Input: part model. Units: mm. Frame: model coordinates. A direction names the side the tool comes from. Give positions to 0.01 mm unless a question says otherwise; leave off trailing zeros. Loops run counter-clockwise (first coordinate to the right, second up) from the corner with the lowest first, then second, coordinate; pieces in that order, holes last.
Autodesk Fusion 360 part; units mm, degrees
sketch "Sketch1" plane through (0, 0, 0) normal (0, 0, 1) x (1, 0, 0)
  circle A0 centre (0, 0) radius 5.25
  circle A1 centre (0, 0) radius 3.1
  circle A2 centre (0, 0) radius 1.85
  circle A3 centre (0, 0) radius 3.4
  circle A4 centre (0, 0) radius 1.55
  dimension "d1" = 10.5
  dimension "d2" = 6.2
  dimension "d3" = 3.7
  dimension "d21" = 0.3
  dimension "d22" = 0.3
extrude "Extrude1" add sketch "Sketch1" along normal blind 9.5 contours A1
extrude "Extrude2" add sketch "Sketch1" along normal blind 2 contours A0 | A3
extrude "Extrude3" add sketch "Sketch1" along normal blind 4 and the other way blind -5 contours A3
chamfer "Chamfer1" distance 0.2 angle 45 2 edges at (-3.1699, -1.2295, 4) (-3.1699, -1.2295, 5)
chamfer "Chamfer2" distance 0.5 angle 45 1 edges at (-1.7248, 0.669, 0)
extrude "Extrude4" add sketch "Sketch1" along normal blind 5 and the other way blind -4 contours A2
chamfer "Chamfer3" distance 0.2 angle 45 2 edges at (-1.4451, 0.5605, 5) (-1.4451, 0.5605, 4)
equation "d2 = OuterRadius"
equation "d3 = InnerRadius"
equation "d21 = NotchThickness"
equation "d22 = NotchThickness"
equation "InnerRadius = 3.7 mm"
equation "OuterRadius = 6.2 mm"
equation "NotchThickness = 0.30 mm"
(1) Reachability of faces 1 (the cylindrical face through (-0.401, 1.806, 2.226)), 2 (the cylindrical face through (1.43, 2.75, 7.22)), 3 (the cylindrical face through (1.43, 2.75, 2.99)) from +Z, -Z, +X, -X, +Y, -Y: full face, straight path, thin tool, end or side. Return the list, or none.
Values follow:
face 1: -Z
face 2: +Z
face 3: none
(2) Cut plane A-A (z = 1.5). Return the cut outline in (x, y), and give its area (3 significant figures).
Values follow:
outline: circle Ø10.5 at (0, 0); hole circle Ø3.7 at (0, 0)
area: 75.8 mm2
(3) Cut plane B-B (x = -4). Return the cut outline in (y, z), and give its area (3 significant figures).
Values follow:
outline: (-3.4, 0) - (3.4, 0) - (3.4, 2) - (-3.4, 2) - close
area: 13.6 mm2
(4) Cut plane C-C (y = 4.75). Return the cut outline in (x, z).
Values follow:
outline: (-2.24, 0) - (2.24, 0) - (2.24, 2) - (-2.24, 2) - close
(5) Mould query, pull axis Y, two halves, no side actions, for faces 4 (the cylindrical face through (-0.401, 1.806, 7.219)), 5 (the cylindrical face through (-0.74, -3.32, 4.5)), 6 (the flat face through (2.3, -1.1, 0)). Classes: +Y half, -Y half, draft (parallel to the pull), parting line (faces both ways), or undercut.
Values follow:
face 4: undercut
face 5: parting line
face 6: draft
(6) Ray query, probe 1 along Y at (x, z) = (0, 2.5); probe 2 along Z at (x, y) = (1, 3); probe 3 along Y at (x, z) = (0, 4.7). Return the intervals inside material, ascending.
Values follow:
probe 1: y = -3.1 to -1.85, 1.85 to 3.1
probe 2: z = 0 to 2, 4 to 5
probe 3: y = -3.4 to -1.55, 1.55 to 3.4
(7) Pin query (flat end, axial travel): pin 1 Ø2 at (x, z) = (4, 4) entering from -Y; pin 2 Ø1.8 at (x, y) = (-0.5, 0) entering from -Z (3 decimals); pin 3 Ø5 at (y, z) = (3, 5) entering from -X; pin 4 Ø2 at (y, z) = (2, 6.5) entering from +X. Return the tip coordinate at first contact, or that it passes through.
Values follow:
pin 1: stops at y = -1.56
pin 2: passes through
pin 3: stops at x = -3.36
pin 4: stops at x = 2.93
(8) Cut plane D-D (z = 8.75). Return the cut outline in (x, y).
Values follow:
outline: circle Ø6.2 at (0, 0); hole circle Ø3.7 at (0, 0)
